The model under review builds one solid part; all positions refer to its coordinate system, in mm. A direction names the side the tool comes from. Round coordinates to 2 decimals unless told otherwise and drop trailing zeros. Write each loop counter-clockwise with the first axis right and the second up, starting at its lowest first coordinate (ties: lowest second). Pieces come first, ordered by that corner, then holes. Notation, with made-up numbers: M 88.5,-8 L 132.5,-8 A9 cw 132.5,-2 Z; hole C 88.25,15.25 d4. An arc over 180 degrees is marked long. One line per item, written item: value. Start each with the question number.
1) Mouldability with a two-part tool opening along X and no side actions: class faces 1 (the face through (-50, 1, 0)), 2 (the face through (-10, 1, 3)), 3 (the face through (11, 1, 20)) as +X half, -X half, draft (parallel to the pull), parting line (faces both ways), or undercut.
2) Take a section at D-D, the plane x = -47. Write out the cut boundary in (y, z).
3) Take a section at B-B, the plane x = 2. Write out the cut boundary in (y, z).
4) Take a section at A-A, the plane x = -16.5. Write out the cut boundary in (y, z), and give its area (3 significant figures).
5) Take a section at C-C, the plane y = 0.75. State how many separate pieces and enclosed holes the cut face has, and give its area (3 significant figures).
6) Wall thickness on probe 1 along Z at (x, y) = (-30, 1.7); probe 2 along Z at (x, y) = (2, 2); probe 3 along X at (y, z) = (2.8, -16): over which ranges is each line inside the solid? List them lowest first.
7) Tool access review of faces 4 (the face through (9, 1, -20)), 5 (the face through (-10, 1, -3)): name each direction out of +Z, -Z, +X, -X, +Y, -Y from which nothing blocks a thin tool from reaching the whole face with its end or side.
from build123d import *

# Parameters (mm, degrees)
BOSS_EXTRUDE1_DEPTH = 3
SKETCH3_R           = 1.75
CUT_EXTRUDE1_DEPTH  = 4
CUT_EXTRUDE2_REACH  = 5
SKETCH4_W           = 20
SKETCH4_H           = 6
FILLET1_R           = 2
CUT_EXTRUDE3_REACH  = 5
SKETCH5_R           = 1.75
CUT_EXTRUDE4_REACH  = 5
SKETCH7_R           = 1.75


with BuildPart() as part:
    # Sketch1 → Boss-Extrude1 (new body)
    with BuildSketch(Plane(origin=(0, 0, 0), x_dir=(1, 0, 0), z_dir=(0, 1, 0))):
        with BuildLine():
            Line((50, -20), (-30, -20))
            ThreePointArc((-30, -20), (-50, 0), (-30, 20))
            Line((-30, 20), (50, 20))
            Line((50, 20), (50, -20))
        make_face()
    extrude(amount=BOSS_EXTRUDE1_DEPTH)

    # Sketch3 → Cut-Extrude1 (cut, through all)
    with BuildSketch(Plane(origin=(0, 3, 0), x_dir=(1, 0, 0), z_dir=(0, 1, 0))):
        with Locations((-30, 10)):
            Circle(SKETCH3_R)
        with Locations((-30, -10)):
            Circle(SKETCH3_R)
    extrude(amount=-CUT_EXTRUDE1_DEPTH, mode=Mode.SUBTRACT)

    # Sketch4 → Cut-Extrude2 (cut, up to next)
    with BuildSketch(Plane.XZ, mode=Mode.PRIVATE) as cut_extrude2_sk1:
        with Locations((-10, 0)):
            Rectangle(SKETCH4_W, SKETCH4_H)
    cut_extrude2_tool1 = extrude(cut_extrude2_sk1.sketch, amount=-CUT_EXTRUDE2_REACH, mode=Mode.PRIVATE) & part.part
    add(cut_extrude2_tool1.solids().sort_by_distance((-10, 0, 0))[0], mode=Mode.SUBTRACT)

    # Fillet1
    fillet1_edges = [part.edges().sort_by_distance(p)[0] for p in [
        (-20, 1.5, -3),
        (-20, 1.5, 3),
        (0, 1.5, 3),
        (0, 1.5, -3),
    ]]
    fillet(fillet1_edges, radius=FILLET1_R)

    # Sketch5 → Cut-Extrude3 (cut, up to next)
    with BuildSketch(Plane.XZ, mode=Mode.PRIVATE) as cut_extrude3_sk1:
        with Locations((-21.5, -14.722431864)):
            Circle(SKETCH5_R)
    cut_extrude3_tool1 = extrude(cut_extrude3_sk1.sketch, amount=-CUT_EXTRUDE3_REACH, mode=Mode.PRIVATE) & part.part
    add(cut_extrude3_tool1.solids().sort_by_distance((-21.5, 0, -14.722432))[0], mode=Mode.SUBTRACT)
    # Sketch5 → Cut-Extrude3 (cut, up to next)
    with BuildSketch(Plane.XZ, mode=Mode.PRIVATE) as cut_extrude3_sk2:
        with Locations((-21.5, 14.722431864)):
            Circle(SKETCH5_R)
    cut_extrude3_tool2 = extrude(cut_extrude3_sk2.sketch, amount=-CUT_EXTRUDE3_REACH, mode=Mode.PRIVATE) & part.part
    add(cut_extrude3_tool2.solids().sort_by_distance((-21.5, 0, 14.722432))[0], mode=Mode.SUBTRACT)
    # Sketch5 → Cut-Extrude3 (cut, up to next)
    with BuildSketch(Plane.XZ, mode=Mode.PRIVATE) as cut_extrude3_sk3:
        with Locations((-47, 0)):
            Circle(SKETCH5_R)
    cut_extrude3_tool3 = extrude(cut_extrude3_sk3.sketch, amount=-CUT_EXTRUDE3_REACH, mode=Mode.PRIVATE) & part.part
    add(cut_extrude3_tool3.solids().sort_by_distance((-47, 0, 0))[0], mode=Mode.SUBTRACT)

    # Sketch7 → Cut-Extrude4 (cut, up to next)
    with BuildSketch(Plane.XZ, mode=Mode.PRIVATE) as cut_extrude4_sk1:
        with Locations((2, 12)):
            Circle(SKETCH7_R)
    cut_extrude4_tool1 = extrude(cut_extrude4_sk1.sketch, amount=-CUT_EXTRUDE4_REACH, mode=Mode.PRIVATE) & part.part
    add(cut_extrude4_tool1.solids().sort_by_distance((2, 0, 12))[0], mode=Mode.SUBTRACT)
    # Sketch7 → Cut-Extrude4 (cut, up to next)
    with BuildSketch(Plane.XZ, mode=Mode.PRIVATE) as cut_extrude4_sk2:
        with Locations((2, -12)):
            Circle(SKETCH7_R)
    cut_extrude4_tool2 = extrude(cut_extrude4_sk2.sketch, amount=-CUT_EXTRUDE4_REACH, mode=Mode.PRIVATE) & part.part
    add(cut_extrude4_tool2.solids().sort_by_distance((2, 0, -12))[0], mode=Mode.SUBTRACT)


solid = part.part
Checked values:
1. face 1: -X half
1. face 2: undercut
1. face 3: draft
2. outline: M 0,-10.54 L 3,-10.54 L 3,-1.75 L 0,-1.75 Z; M 0,1.75 L 3,1.75 L 3,10.54 L 0,10.54 Z
3. outline: M 0,-20 L 3,-20 L 3,-13.75 L 0,-13.75 Z; M 0,-10.25 L 3,-10.25 L 3,10.25 L 0,10.25 Z; M 0,13.75 L 3,13.75 L 3,20 L 0,20 Z
4. outline: M 0,-20 L 3,-20 L 3,-3 L 0,-3 Z; M 0,3 L 3,3 L 3,20 L 0,20 Z
4. area: 102 mm2
5. separate pieces: 1
5. enclosed holes: 8
5. area: 3,640 mm2
6. probe 1: z = -20 to -11.75, -8.25 to 8.25, 11.75 to 20
6. probe 2: z = -20 to -13.75, -10.25 to 10.25, 13.75 to 20
6. probe 3: x = -42 to -22.7, -20.3 to 50
7. face 4: -Z, +X, -X, +Y, -Y
7. face 5: +Y, -Y
